The listing builds one solid part. Answer for the finished solid, in the listing's coordinates (mm). A direction names the side the tool comes from. Coordinates: 2 decimals unless noted, no trailing zeros. Write each loop counter-clockwise with the first axis right and the second up, starting at its lowest first coordinate (ties: lowest second). Pieces come first, ordered by that corner, then holes.
from build123d import *

# Parameters (mm, degrees)
SKETCH2_W          = 1.587498625
SKETCH2_H          = 34.925
SKETCH3_W          = 7.264393708
SKETCH3_H          = 7.264393708
CUT_EXTRUDE1_DEPTH = 1.14299901


with BuildPart() as part:
    # Sketch1 → Base-Revolve (revolve)
    with BuildSketch(Plane.XY, mode=Mode.PRIVATE) as base_revolve_sk:
        Polygon((0, 0), (3.30199714, 0), (3.30199714, 1.332469781), (2.346557647, 1.77799846), (2.252695341, 1.77799846), (2.229229765, 1.684136154), (0, 1.684136154), align=None)
    revolve(base_revolve_sk.sketch.rotate(Axis((0, 0, 0), (0, 1, 0)), 90), axis=Axis((0, 0, 0), (0, 1, 0)))

    # Sketch2 → Boss-Revolve1 (revolve)
    with BuildSketch(Plane.XY, mode=Mode.PRIVATE) as boss_revolve1_sk:
        with Locations((0.793749313, -17.4625)):
            Rectangle(SKETCH2_W, SKETCH2_H)
    revolve(boss_revolve1_sk.sketch.rotate(Axis((0, 0, 0), (0, 1, 0)), 90), axis=Axis((0, 0, 0), (0, 1, 0)))

    # Sketch3 → Cut-Extrude1 (cut)
    with BuildSketch(Plane(origin=(0, 1.77799846, 0), x_dir=(-1, 0, 0), z_dir=(0, 1, 0))):
        Rectangle(SKETCH3_W, SKETCH3_H)
        Polygon((2.387597932, 1.378480068), (6.25e-07, 2.756960497), (-2.387597307, 1.378481151), (-2.387598557, -1.378478985), (-1.876e-06, -2.756960497), (2.387596681, -1.378482234), align=None, mode=Mode.SUBTRACT)
    extrude(amount=-CUT_EXTRUDE1_DEPTH, mode=Mode.SUBTRACT)


solid = part.part
1. Find the intervals of material crossed by L1, parallel to Y at x = 2.5, z = -0.75 (3 decimals); L2, parallel to Y at x = -0.75, z = -1.5; L3, parallel to Z at x = 1.25, y = -8, in increasing order.
Results found:
L1: y = 0 to 0.635
L2: y = 0 to 1.68
L3: z = -0.98 to 0.98
2. Flat-ended cylindrical pins translate along their axes: P1, Ø1.2, axis at y = 1.5, z = -0.5, coming from the -X side; P2, Ø1.5, axis at x = -0.5, z = 0, coming from the +Y side. Find the tip coordinate at first contact, or state that the pin passes through.
Results found:
P1: stops at x = -2.39
P2: stops at y = 1.68
3. A tool of negligible diameter and unlimited length cuts with its end or side. For faces 1 (the flat face through (-1.21, 1.2, 2.06)), 2 (the flat face through (1.177, 1.205, 2.077)), 3 (the flat face through (-1.177, 1.205, -2.077)), from which of +Z, -Z, +X, -X, +Y, -Y can it reach the whole face along a straight path? Write none if from no direction.
Results found:
face 1: +Z, -X, +Y
face 2: +Z, +X, +Y
face 3: -Z, -X, +Y
4. Section B-B on y = -27 is taken. Give the vertices of the cut face in (x, z) (1 decimal), then the cut area to 3 significant figures.
Results found:
outline: circle Ø3.2 at (0, 0)
area: 7.92 mm2
5. For a pull along Z with two mould halves and no side action, classify faces 4 (the flat face through (0, 1.684, 0)), 5 (the flat face through (1.21, 1.2, -2.06)), 6 (the cylindrical face through (-0.477, -17.218, -1.514)) as pulls with the +Z half, pulls with the -Z half, needs draft (parallel to the pull), parting line crosses it, or undercut.
Results found:
face 4: undercut
face 5: pulls with the -Z half
face 6: parting line crosses it
